from build123d import *

# Parameters (mm, degrees)
SKETCH1_W           = 203.2
SKETCH1_H           = 127
BOSS_EXTRUDE1_DEPTH = 127
SHELL1_T            = -6.35
SKETCH2_R           = 2.38125
CUT_EXTRUDE1_DEPTH  = 204.2
SKETCH4_R           = 3.794312019
CUT_EXTRUDE3_DEPTH  = 23.368


with BuildPart() as part:
    # Sketch1 → Boss-Extrude1 (new body)
    with BuildSketch(Plane(origin=(0, 0, 0), x_dir=(1, 0, 0), z_dir=(0, 1, 0))):
        with Locations((101.6, 63.5)):
            Rectangle(SKETCH1_W, SKETCH1_H)
    extrude(amount=BOSS_EXTRUDE1_DEPTH)

    # Shell1
    shell1_openings = [part.faces().sort_by_distance(p)[0] for p in [
        (101.6, 63.5, 0),
    ]]
    offset(amount=SHELL1_T, openings=shell1_openings, kind=Kind.INTERSECTION)

    # Sketch2 → Cut-Extrude1 (cut, through all)
    with BuildSketch(Plane(origin=(203.2, 0, 0), x_dir=(0, 0, -1), z_dir=(1, 0, 0))):
        with Locations((63.5, 63.5)):
            Circle(SKETCH2_R)
    extrude(amount=-CUT_EXTRUDE1_DEPTH, mode=Mode.SUBTRACT)

    # Sketch4 → Cut-Extrude3 (cut)
    with BuildSketch(Plane(origin=(0, 127, 0), x_dir=(1, 0, 0), z_dir=(0, 1, 0))):
        with Locations((73.037262301, 63.5)):
            Circle(SKETCH4_R)
        with Locations((130.162737699, 63.5)):
            Circle(SKETCH4_R)
    extrude(amount=-CUT_EXTRUDE3_DEPTH, mode=Mode.SUBTRACT)


solid = part.part
Geometry check sheet. Reference: the model listing, model coordinates, mm. A direction names the side the tool comes from. Round coordinates to 2 decimals unless told otherwise and drop trailing zeros. Write each loop counter-clockwise with the first axis right and the second up, starting at its lowest first coordinate (ties: lowest second). Pieces come first, ordered by that corner, then holes.
Item 1: Section check D-D (y = 63.5). Record the boundary of the cut face in (x, z).
Determined:
outline: (0, -127) - (203.2, -127) - (203.2, -65.88) - (196.85, -65.88) - (196.85, -120.65) - (6.35, -120.65) - (6.35, -65.88) - (0, -65.88) - close; (0, -61.12) - (6.35, -61.12) - (6.35, 0) - (0, 0) - close; (196.85, -61.12) - (203.2, -61.12) - (203.2, 0) - (196.85, 0) - close
Item 2: Section check B-B (z = -16.5). Record the boundary of the cut face in (x, y), plus the area to 3 significant figures.
Determined:
outline: (0, 0) - (203.2, 0) - (203.2, 127) - (0, 127) - close; hole (6.35, 6.35) - (196.85, 6.35) - (196.85, 120.65) - (6.35, 120.65) - close
area: 4,030 mm2
Item 3: Section check C-C (x = 106). Record the boundary of the cut face in (y, z).
Determined:
outline: (0, -127) - (127, -127) - (127, 0) - (120.65, 0) - (120.65, -120.65) - (6.35, -120.65) - (6.35, 0) - (0, 0) - close
Item 4: Section check A-A (z = -63.5). Record the boundary of the cut face in (x, y).
Determined:
outline: (0, 0) - (203.2, 0) - (203.2, 61.12) - (196.85, 61.12) - (196.85, 6.35) - (6.35, 6.35) - (6.35, 61.12) - (0, 61.12) - close; (0, 65.88) - (6.35, 65.88) - (6.35, 120.65) - (69.24, 120.65) - (69.24, 127) - (0, 127) - close; (76.83, 120.65) - (126.37, 120.65) - (126.37, 127) - (76.83, 127) - close; (133.96, 120.65) - (196.85, 120.65) - (196.85, 65.88) - (203.2, 65.88) - (203.2, 127) - (133.96, 127) - close
Item 5: Go/stop test with a flat-tipped pin: pin 1 Ø12 at (x, y) = (100, 105) entering from +Z. Record where the tip stops, or that it passes through.
Determined:
pin 1: stops at z = -120.65
Item 6: Mould release check, pull along Z, two halves, no side actions. Record for faces 1 (the face through (100, 63, -120.65)), 2 (the face through (76.656, 123.869, -64.64)), 3 (the face through (196.85, 63, -59)): +Z half, -Z half, draft (parallel to the pull), parting line (faces both ways), or undercut.
Determined:
face 1: +Z half
face 2: undercut
face 3: draft
Item 7: Access from +Z, -Z, +X, -X, +Y, -Y to the whole of each face (thin tool, end or side, straight path). Record for faces 4 (the face through (100, 0, -64)), 5 (the face through (100, 120.65, -61)), 6 (the face through (126.372, 123.869, -63.667)).
Determined:
face 4: +Z, -Z, +X, -X, -Y
face 5: +Z
face 6: +Y
Item 8: Material ranges on line 1 along X through (y, z) = (123, -63); line 2 along X through (y, z) = (125.75, -63.5); line 3 along X through (y, z) = (10.5, -86), recorded low to high.
Determined:
line 1: x = 0 to 69.28, 76.8 to 126.4, 133.92 to 203.2
line 2: x = 0 to 69.24, 76.83 to 126.37, 133.96 to 203.2
line 3: x = 0 to 6.35, 196.85 to 203.2
